Geometry check sheet. Reference: the model listing, model coordinates, mm. A direction names the side the tool comes from. Round coordinates to 2 decimals unless told otherwise and drop trailing zeros. Order: outer loops, then holes, each group sorted by start corner. A loop starts at its lowest first (then second) coordinate and runs counter-clockwise, first axis right, second up. Notation, with made-up numbers: (-24, 9.5) - (15, 9.5) arc R18 ccw to (15, 23.5) - close; hole circle Ø8 at (5, 63). An arc over 180 degrees is marked (long way). Return JSON: item names as keys, results as strings. Group by question number.
Q1. Sectioned sample at D-D, the plane x = -119. Record the cut outline in (y, z), then the cut area to 3 significant figures.
Q2. Sectioned sample at A-A, the plane x = 8. Record the cut outline in (y, z), then the cut area to 3 significant figures.
Q3. Tool access check on faces 5 (the cylindrical face through (-28.29, 12.11, 23.26)), 6 (the flat face through (-88.825, 10.14, -17.07)), 7 (the cylindrical face through (-39.908, 10.14, 49.747)). Record the directions out of +Z, -Z, +X, -X, +Y, -Y that give a thin tool (end or side, any length) a straight path to the whole face; none if there is none.
Q4. Draft check along Z on faces 1 (the cylindrical face through (-55.5, 10.1, 0.2)), 2 (the cylindrical face through (-129, 10, 0)), 3 (the flat face through (-83.32, 9.86, 28.693)), 4 (the cylindrical face through (28.063, 12.112, 23.129)). Enter one of: pulls with the +Z half, pulls with the -Z half, needs draft (parallel to the pull), parting line crosses it, or undercut.
Q5. Material ranges on line 1 along Z through (x, y) = (-2.5, 16.25); line 2 along X through (y, z) = (2.5, 14); line 3 along X through (y, z) = (13.5, 21.5), recorded low to high.
Q6. Sectioned sample at B-B, the plane z = 0. Give the number of separate pieces and of enclosed holes in the cut face, then the cut area to 3 significant figures.
Q7. Gauge pin test, flat ends, axial feed: pin 1 Ø5 at (x, z) = (10, 35) entering from +Y; pin 2 Ø3 at (x, y) = (-57, 14.5) entering from -Z; pin 3 Ø10 at (x, y) = (50.5, 5.5) entering from +Z. Record the tip position at first contact, or that the pin passes through.
```python
from build123d import *

# Parameters (mm, degrees)
BOSS_EXTRUDE1_DEPTH = 20
SKETCH2_R           = 47.5
SKETCH2_R_2         = 45
CUT_EXTRUDE1_DEPTH  = 1
CUT_EXTRUDE2_DEPTH  = 16
CIRPATTERN1_COUNT   = 4
SKETCH4_R           = 25
CUT_EXTRUDE3_DEPTH  = 21
SKETCH6_R           = 4
CUT_EXTRUDE4_DEPTH  = 21
CUT_EXTRUDE5_DEPTH  = 21
FILLET1_R           = 10
SKETCH9_R           = 4
CUT_EXTRUDE6_DEPTH  = 21


with BuildPart() as part:
    # Sketch1 → Boss-Extrude1 (new body)
    with BuildSketch(Plane(origin=(0, 0, 0), x_dir=(1, 0, 0), z_dir=(0, 1, 0))):
        with BuildLine():
            Line((-40, -50), (40, -50))
            Line((40, -50), (123.413509856, -8.973345572))
            ThreePointArc((123.413509856, -8.973345572), (129, 0), (123.413509856, 8.973345572))
            Line((123.413509856, 8.973345572), (40, 50))
            Line((40, 50), (-40, 50))
            Line((-40, 50), (-123.413509856, 8.973345572))
            ThreePointArc((-123.413509856, 8.973345572), (-129, 0), (-123.413509856, -8.973345572))
            Line((-123.413509856, -8.973345572), (-40, -50))
        make_face()
    extrude(amount=BOSS_EXTRUDE1_DEPTH)

    # Sketch2 → Cut-Extrude1 (cut)
    with BuildSketch(Plane(origin=(0, 20, 0), x_dir=(1, 0, 0), z_dir=(0, 1, 0))):
        with Locations(Location((0, 0, 0), (0, 0, 270))):  # turned: the seam where the file's is
            Circle(SKETCH2_R)
        with Locations(Location((0, 0, 0), (0, 0, 270))):  # turned: the seam where the file's is
            Circle(SKETCH2_R_2, mode=Mode.SUBTRACT)
    extrude(amount=-CUT_EXTRUDE1_DEPTH, mode=Mode.SUBTRACT)

    # Sketch3 → Cut-Extrude2 (cut)
    with BuildSketch(Plane(origin=(0, 20, 0), x_dir=(1, 0, 0), z_dir=(0, 1, 0))):
        with BuildLine():
            ThreePointArc((36.373066959, -21), (42, 0), (36.373066959, 21))
            ThreePointArc((36.373066959, 21), (28.176914536, 23.196152423), (25.980762114, 15))
            ThreePointArc((25.980762114, 15), (30, 0), (25.980762114, -15))
            ThreePointArc((25.980762114, -15), (28.176914536, -23.196152423), (36.373066959, -21))
        make_face()
    cut_extrude2 = extrude(amount=-CUT_EXTRUDE2_DEPTH, mode=Mode.SUBTRACT)

    # CirPattern1: Cut-Extrude2 ×4 about axis
    cirpattern1_axis = Axis((0, 0, 0), (0, 1, 0))
    for i in range(1, CIRPATTERN1_COUNT):
        add(cut_extrude2.rotate(cirpattern1_axis, i * 360 / CIRPATTERN1_COUNT), mode=Mode.SUBTRACT)

    # Sketch4 → Cut-Extrude3 (cut, through all)
    with BuildSketch(Plane(origin=(0, 20, 0), x_dir=(1, 0, 0), z_dir=(0, 1, 0))):
        with Locations(Location((0, 0, 0), (0, 0, 270))):  # turned: the seam where the file's is
            Circle(SKETCH4_R)
    extrude(amount=-CUT_EXTRUDE3_DEPTH, mode=Mode.SUBTRACT)

    # Sketch6 → Cut-Extrude4 (cut, through all)
    with BuildSketch(Plane(origin=(0, 20, 0), x_dir=(1, 0, 0), z_dir=(0, 1, 0))):
        with Locations(Location((-119, 0, 0), (0, 0, 270))):  # turned: the seam where the file's is
            Circle(SKETCH6_R)
        with Locations(Location((119, 0, 0), (0, 0, 270))):  # turned: the seam where the file's is
            Circle(SKETCH6_R)
    extrude(amount=-CUT_EXTRUDE4_DEPTH, mode=Mode.SUBTRACT)

    # Sketch8 → Cut-Extrude5 (cut, through all)
    with BuildSketch(Plane(origin=(0, 20, 0), x_dir=(1, 0, 0), z_dir=(0, 1, 0))):
        with BuildLine():
            Line((-67.173638652, 27.719444727), (-111.090654796, 6.119007963))
            ThreePointArc((-111.090654796, 6.119007963), (-109, 0), (-111.090654796, -6.119007963))
            Line((-111.090654796, -6.119007963), (-67.173638652, -27.719444727))
            ThreePointArc((-67.173638652, -27.719444727), (-56.30285419, -26.381778867), (-53.178429743, -15.884099284))
            ThreePointArc((-53.178429743, -15.884099284), (-55.5, 0), (-53.178429743, 15.884099284))
            ThreePointArc((-53.178429743, 15.884099284), (-56.30285419, 26.381778867), (-67.173638652, 27.719444727))
        make_face()
    cut_extrude5 = extrude(amount=-CUT_EXTRUDE5_DEPTH, mode=Mode.SUBTRACT)

    # Mirror1: Cut-Extrude5 across plane
    add(cut_extrude5.mirror(Plane(origin=(0, 0, 0), x_dir=(0, 0, 1), z_dir=(1, 0, 0))), mode=Mode.SUBTRACT)

    # Fillet1
    fillet1_edges = [part.edges().sort_by_distance(p)[0] for p in [
        (40, 10, 50),
        (-40, 10, 50),
        (-40, 10, -50),
        (40, 10, -50),
    ]]
    fillet(fillet1_edges, radius=FILLET1_R)

    # Sketch9 → Cut-Extrude6 (cut, through all)
    with BuildSketch(Plane(origin=(0, 20, 0), x_dir=(1, 0, 0), z_dir=(0, 1, 0))):
        with Locations(Location((-37.673836784, 40, 0), (0, 0, 270))):  # turned: the seam where the file's is
            Circle(SKETCH9_R)
        with Locations(Location((37.673836784, 40, 0), (0, 0, 270))):  # turned: the seam where the file's is
            Circle(SKETCH9_R)
        with Locations(Location((-37.673836784, -40, 0), (0, 0, 270))):  # turned: the seam where the file's is
            Circle(SKETCH9_R)
        with Locations(Location((37.673836784, -40, 0), (0, 0, 270))):  # turned: the seam where the file's is
            Circle(SKETCH9_R)
    extrude(amount=-CUT_EXTRUDE6_DEPTH, mode=Mode.SUBTRACT)


solid = part.part
```
Reply:
{
 "1": {"outline": "(0, -11.14) - (20, -11.14) - (20, -4) - (0, -4) - close; (0, 4) - (20, 4) - (20, 11.14) - (0, 11.14) - close", "area": "286 mm^2"},
 "2": {"outline": "(0, -50) - (20, -50) - (20, -46.82) - (19, -46.82) - (19, -44.28) - (20, -44.28) - (20, -41.23) - (4, -41.23) - (4, -28.91) - (20, -28.91) - (20, -23.69) - (0, -23.69) - close; (0, 23.69) - (20, 23.69) - (20, 28.91) - (4, 28.91) - (4, 41.23) - (20, 41.23) - (20, 44.28) - (19, 44.28) - (19, 46.82) - (20, 46.82) - (20, 50) - (0, 50) - close", "area": "653 mm^2"},
 "3": {"face 5": "+Y", "face 6": "+Y, -Y", "face 7": "+Z, -X, +Y, -Y"},
 "4": {"face 1": "undercut", "face 2": "parting line crosses it", "face 3": "pulls with the +Z half", "face 4": "undercut"},
 "5": {"line 1": "-50 to -41.93, -29.9 to -24.87, 24.87 to 29.9, 41.93 to 50", "line 2": "-113.19 to -95.07, -53.71 to -20.71, 20.71 to 53.71, 95.07 to 113.19", "line 3": "-97.94 to -79.82, -53.15 to -36.05, -26.3 to -12.76, 12.76 to 26.3, 36.05 to 53.15, 79.82 to 97.94"},
 "6": {"separate pieces": "6", "enclosed holes": "0", "area": "1,310 mm^2"},
 "7": {"pin 1": "y = 4", "pin 2": "z = -42.38", "pin 3": "z = 47.29"}
}
